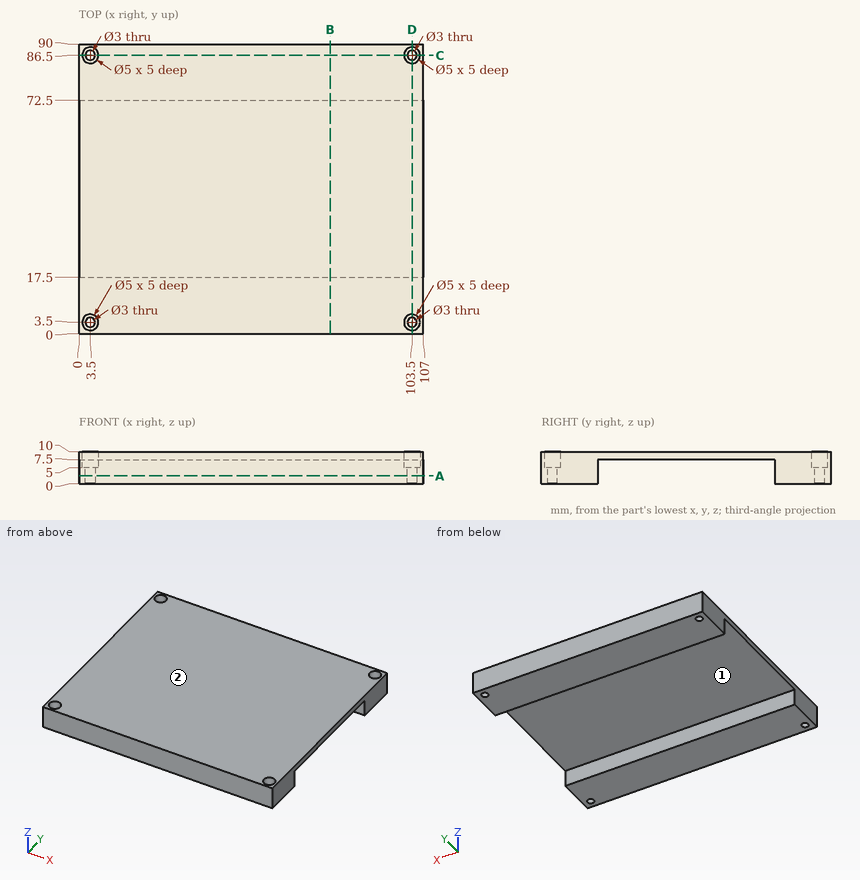
Answer from the drawing. Dimensions are ordinates in mm from the lowest x, y and z of the part. A direction names the side the tool comes from. Give positions to 0.01 mm unless a question says otherwise; leave off trailing zeros. Loops run counter-clockwise (first coordinate to the right, second up) from the corner with the lowest first, then second, coordinate; pieces in that order, holes last. Notation, with made-up numbers: M -28.75,-21.75 L 18.25,-21.75 A33 cw 18.25,9.25 Z; hole C 43,22.5 d9. An arc over 180 degrees is marked long. One line per item, written item: value.
Q1. A cutting plane is placed at D-D on x = 103.5. Determine the outline of the cut face in (y, z).
Working result:
outline: M 0,0 L 2,0 L 2,5 L 1,5 L 1,10 L 0,10 Z; M 5,0 L 17.5,0 L 17.5,7.5 L 72.5,7.5 L 72.5,0 L 85,0 L 85,5 L 84,5 L 84,10 L 6,10 L 6,5 L 5,5 Z; M 88,0 L 90,0 L 90,10 L 89,10 L 89,5 L 88,5 Z
Q2. For the marked faces 1 and 2, determine the directions among +Z, -Z, +X, -X, +Y, -Y from which every point of the face is accessible in a straight line to the end or side of a thin tool.
Working result:
face 1: -Z, +X, -X
face 2: +Z, +X, -X, +Y, -Y
Q3. A cutting plane is placed at C-C on y = 86.5. Determine the outline of the cut face in (x, z).
Working result:
outline: M 0,0 L 2,0 L 2,5 L 1,5 L 1,10 L 0,10 Z; M 5,0 L 102,0 L 102,5 L 101,5 L 101,10 L 6,10 L 6,5 L 5,5 Z; M 105,0 L 107,0 L 107,10 L 106,10 L 106,5 L 105,5 Z
Q4. Flat-ended cylindrical pins translate along their axes: P1, Ø4, axis at x = 103.5, y = 3.5, coming from the +Z side; P2, Ø12, axis at x = 83.5, y = 42, coming from the -Z side. Find the tip coordinate at first contact, or state that the pin passes through.
Working result:
P1: stops at z = 5
P2: stops at z = 7.5
Q5. A cutting plane is placed at A-A on z = 2.5. Determine the outline of the cut face in (x, y), then the cut area to 3 significant figures.
Working result:
outline: M 0,0 L 107,0 L 107,17.5 L 0,17.5 Z; M 0,72.5 L 107,72.5 L 107,90 L 0,90 Z; hole C 3.5,3.5 d3; hole C 3.5,86.5 d3; hole C 103.5,3.5 d3; hole C 103.5,86.5 d3
area: 3,720 mm^2
Q6. Find the intervals of material crossed by line 1 (X direction, y = 86.5, z = 1.95); line 2 (Y direction, x = 3.5, z = 2.8); line 3 (Y direction, x = 3.5, z = 8.2), in increasing order. Write a range as from..to.
Working result:
line 1: x = 0..2, 5..102, 105..107
line 2: y = 0..2, 5..17.5, 72.5..85, 88..90
line 3: y = 0..1, 6..84, 89..90
Q7. A cutting plane is placed at B-B on x = 78. Determine the outline of the cut face in (y, z).
Working result:
outline: M 0,0 L 17.5,0 L 17.5,7.5 L 72.5,7.5 L 72.5,0 L 90,0 L 90,10 L 0,10 Z
